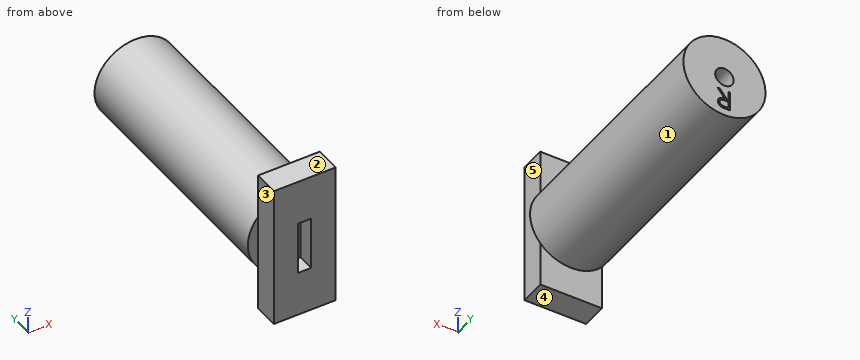
from build123d import *

# Parameters (mm, degrees)
SKETCH1_R           = 10
BOSS_EXTRUDE1_DEPTH = 4
SKETCH2_R           = 10
SKETCH2_R_2         = 8
SKETCH2_R_3         = 3.5
BOSS_EXTRUDE2_DEPTH = 52
SKETCH3_R           = 10
BOSS_EXTRUDE3_DEPTH = 4
CUT_EXTRUDE1_DEPTH  = 2
SKETCH5_R           = 2.25
CUT_EXTRUDE2_DEPTH  = 50
SKETCH6_W           = 15
SKETCH6_H           = 35
BOSS_EXTRUDE4_DEPTH = 6.18
SKETCH7_W           = 3.18
SKETCH7_H           = 13
CUT_EXTRUDE3_DEPTH  = 4.18


with BuildPart() as part:
    # Sketch1 → Boss-Extrude1 (new body)
    with BuildSketch(Plane(origin=(0, 0, 0), x_dir=(1, 0, 0), z_dir=(0, 1, 0))):
        with Locations(Location((0, 0, 0), (0, 0, 270))):
            Circle(SKETCH1_R)
    extrude(amount=BOSS_EXTRUDE1_DEPTH)

    # Sketch2 → Boss-Extrude2 (add)
    # profile 1 of 2: a face of its own
    with BuildSketch(Plane(origin=(0, 4, 0), x_dir=(1, 0, 0), z_dir=(0, 1, 0))):
        with Locations(Location((0, 0, 0), (0, 0, 270))):
            Circle(SKETCH2_R)
        with Locations(Location((0, 0, 0), (0, 0, 90))):
            Circle(SKETCH2_R_2, mode=Mode.SUBTRACT)
    # profile 2 of 2: a face of its own
    with BuildSketch(Plane(origin=(0, 4, 0), x_dir=(1, 0, 0), z_dir=(0, 1, 0))):
        with Locations(Location((0, 0, 0), (0, 0, 90))):
            Circle(SKETCH2_R_3)
    extrude(amount=BOSS_EXTRUDE2_DEPTH)

    # Sketch3 → Boss-Extrude3 (add)
    with BuildSketch(Plane(origin=(0, 56, 0), x_dir=(1, 0, 0), z_dir=(0, 1, 0))):
        with Locations(Location((0, 0, 0), (0, 0, 270))):
            Circle(SKETCH3_R)
    extrude(amount=BOSS_EXTRUDE3_DEPTH)

    # Sketch4 → Cut-Extrude1 (cut)
    with BuildSketch(Plane(origin=(0, 60, 0), x_dir=(1, 0, 0), z_dir=(0, 1, 0))):
        with BuildLine():
            Line((-1.404326923, 8.220249015), (-0.451254507, 8.220249015))
            add(Edge.make_bspline(
                [(-0.451254507, 8.220249015), (-0.387653186, 8.220037307), (-0.265531604, 8.219630804), (-0.090580118, 8.217364176), (0.068388182, 8.210867642), (0.211290178, 8.205277034), (0.338123247, 8.195082643), (0.449276311, 8.185339048), (0.544237428, 8.172584174), (0.601721961, 8.16073858), (0.627749399, 8.155375217)],
                knots=[0, 0, 0, 0, 1.410062039, 2.707475311, 3.878576406, 4.937260626, 5.877586885, 6.699081471, 7.410979367, 8, 8, 8, 8], degree=3))
            add(Edge.make_bspline(
                [(0.627749399, 8.155375217), (0.662592698, 8.146766297), (0.731535995, 8.129732108), (0.830800192, 8.093728152), (0.925389325, 8.052063591), (1.014910479, 8.003127243), (1.098915252, 7.946555846), (1.178269811, 7.883326008), (1.253334245, 7.813783703), (1.32107282, 7.73617558), (1.384943458, 7.654755186), (1.438812268, 7.56671186), (1.485248657, 7.474643853), (1.522219967, 7.377614831), (1.551989638, 7.276565777), (1.572980343, 7.170581378), (1.585568566, 7.06014448), (1.586850162, 6.984818183), (1.5875, 6.946623714)],
                knots=[0, 0, 0, 0, 1.027469482, 2.033020251, 3.019912614, 3.986113645, 4.951240523, 5.91722682, 6.890402269, 7.87763091, 8.8651537, 9.85103654, 10.82876324, 11.815024772, 12.821070561, 13.842952187, 14.906261191, 16, 16, 16, 16], degree=3))
            add(Edge.make_bspline(
                [(1.5875, 6.946623714), (1.585501113, 6.883166661), (1.581600768, 6.759345515), (1.545235537, 6.579648387), (1.485668201, 6.412022927), (1.40358544, 6.256680195), (1.299056082, 6.116648209), (1.17342842, 5.993652625), (1.02663237, 5.890728316), (0.889976765, 5.819355035), (0.769262086, 5.773644684), (0.669884614, 5.741482353), (0.56148062, 5.716633036), (0.445088747, 5.694371571), (0.32022463, 5.677564444), (0.187187541, 5.665254614), (0.045882599, 5.657561069), (-0.051189492, 5.656415341), (-0.101126803, 5.655825938)],
                knots=[0, 0, 0, 0, 1.260483769, 2.459530307, 3.627416485, 4.787058657, 5.939039949, 7.08810263, 8.267026773, 9.491475466, 10.141966685, 10.831826277, 11.566392101, 12.351337768, 13.187381173, 14.07005841, 15.007169909, 16, 16, 16, 16], degree=3))
            Line((-0.101126803, 5.655825938), (1.648557692, 3.457749015))
            Line((1.648557692, 3.457749015), (1.120027043, 3.457749015))
            Line((1.120027043, 3.457749015), (-0.629657452, 5.655825938))
            Line((-0.629657452, 5.655825938), (-0.976923077, 5.655825938))
            Line((-0.976923077, 5.655825938), (-0.976923077, 3.457749015))
            Line((-0.976923077, 3.457749015), (-1.404326923, 3.457749015))
            Line((-1.404326923, 3.457749015), (-1.404326923, 8.220249015))
        make_face()
        with BuildLine():
            Line((-0.976923077, 7.731787476), (-0.976923077, 6.144287476))
            Line((-0.976923077, 6.144287476), (-0.104942909, 6.137609291))
            add(Edge.make_bspline(
                [(-0.104942909, 6.137609291), (-0.064230284, 6.13759128), (0.014682377, 6.137556369), (0.128847211, 6.142990757), (0.235146363, 6.149172915), (0.333173243, 6.158628989), (0.422971644, 6.170815644), (0.504496681, 6.186059705), (0.577881434, 6.203819833), (0.663468374, 6.231308474), (0.759040225, 6.27485952), (0.862905533, 6.338221859), (0.951355143, 6.417917696), (1.026082663, 6.509049435), (1.08613021, 6.60924733), (1.128464827, 6.717310318), (1.15532865, 6.830510314), (1.158497136, 6.908313383), (1.160096154, 6.947577741)],
                knots=[0, 0, 0, 0, 1.146690395, 2.22261258, 3.21895312, 4.145990853, 4.996080663, 5.770904154, 6.481378293, 7.121626537, 8.300444488, 9.431385265, 10.535395872, 11.636531494, 12.74115979, 13.810798291, 14.895190096, 16, 16, 16, 16], degree=3))
            add(Edge.make_bspline(
                [(1.160096154, 6.947577741), (1.158460411, 6.985877186), (1.155218964, 7.061772711), (1.128754747, 7.172883074), (1.084001696, 7.277749174), (1.023691794, 7.37594442), (0.950214372, 7.46507901), (0.86405692, 7.541343172), (0.767575208, 7.60427548), (0.677399041, 7.644490547), (0.596798202, 7.66914649), (0.526817129, 7.686497181), (0.447744011, 7.700436976), (0.359194905, 7.711605802), (0.261547829, 7.721205566), (0.15430905, 7.727671379), (0.038190074, 7.731500244), (-0.042292, 7.731689504), (-0.083954327, 7.731787476)],
                knots=[0, 0, 0, 0, 1.101028733, 2.181837193, 3.264309656, 4.369019818, 5.486613113, 6.575447106, 7.666700264, 8.788928104, 9.402425223, 10.0903467, 10.862060571, 11.710948788, 12.657782767, 13.684531032, 14.801375019, 16, 16, 16, 16], degree=3))
            Line((-0.083954327, 7.731787476), (-0.976923077, 7.731787476))
        make_face(mode=Mode.SUBTRACT)
    extrude(amount=-CUT_EXTRUDE1_DEPTH, mode=Mode.SUBTRACT)

    # Sketch5 → Cut-Extrude2 (cut)
    with BuildSketch(Plane(origin=(0, 60, 0), x_dir=(1, 0, 0), z_dir=(0, 1, 0))):
        with Locations(Location((0, 0, 0), (0, 0, 270))):
            Circle(SKETCH5_R)
    extrude(amount=-CUT_EXTRUDE2_DEPTH, mode=Mode.SUBTRACT)

    # Sketch6 → Boss-Extrude4 (add)
    with BuildSketch(Plane.XZ):
        Rectangle(SKETCH6_W, SKETCH6_H)
    extrude(amount=BOSS_EXTRUDE4_DEPTH)

    # Sketch7 → Cut-Extrude3 (cut)
    with BuildSketch(Plane.XZ.offset(6.18)):
        Rectangle(SKETCH7_W, SKETCH7_H)
    extrude(amount=-CUT_EXTRUDE3_DEPTH, mode=Mode.SUBTRACT)


solid = part.part
Check sheet for the modelled part. Datum: model origin and axes. Units: mm. Face numbers are marked on the shaded views. A direction names the side the tool comes from. Coordinates: 2 decimals unless noted, no trailing zeros. Write each loop counter-clockwise with the first axis right and the second up, starting at its lowest first coordinate (ties: lowest second). Pieces come first, ordered by that corner, then holes. Notation, with made-up numbers: M 22.5,82 L 69.5,82 A12 cw 69.5,88 Z; hole C 29.25,86.5 d5. An arc over 180 degrees is marked long. Answer as CSV lines item,"result".
Q1. Set-up check for the marked faces 4 and 5: record each of +Z, -Z, +X, -X, +Y, -Y from which the full face is reachable in a straight line by a thin tool's end or side.
Check result:
face 4,"-Z, +X, -X, +Y, -Y"
face 5,"+Z, -Z, +X, -Y"
Q2. Cross-section at C-C (y = 5). Record the boundary of the cut face in (x, z).
Check result:
outline,"C 0,0 d20; C 0,0 d7; hole C 0,0 d16"
Q3. Go/stop test with flat-tipped pins: pin 1 (3 mm diameter, centred on x = -3.5, z = 12.5, fed in from +Y); pin 2 (2 mm diameter, centred on x = 1, z = 0.5, fed in from +Y); pin 3 (2 mm diameter, centred on y = 59, z = -4.5, fed in from -X); pin 4 (1.5 mm diameter, centred on y = 34, z = 12, fed in from -X). Record where each tip stops, or that it passes through.
Check result:
pin 1,"y = 0"
pin 2,"y = 10"
pin 3,"x = -9.37"
pin 4,"through"
Q4. Material ranges on probe 1 along X at (y, z) = (34, 0); probe 2 along Y at (x, z) = (2.25, -5); probe 3 along Y at (x, z) = (0.5, -5), recorded low to high. Write a range as from..to.
Check result:
probe 1,"-10..-8, -3.5..-2.25, 2.25..3.5, 8..10"
probe 2,"-6.18..4, 56..60"
probe 3,"-2..4, 56..60"
Q5. Cross-section at A-A (z = 0). Record the boundary of the cut face in (x, y).
Check result:
outline,"M -10,0 L -7.5,0 L -7.5,-6.18 L -1.59,-6.18 L -1.59,-2 L 1.59,-2 L 1.59,-6.18 L 7.5,-6.18 L 7.5,0 L 10,0 L 10,60 L 2.25,60 L 2.25,10 L -2.25,10 L -2.25,60 L -10,60 Z; hole M -8,4 L -3.5,4 L -3.5,56 L -8,56 Z; hole M 3.5,4 L 8,4 L 8,56 L 3.5,56 Z"
Q6. Mould release check, pull along Z, two halves, no side actions. Record for the marked faces 1, 2 and 3: released by +Z, released by -Z, zero draft, split by the parting line, or undercut.
Check result:
face 1,"split by the parting line"
face 2,"released by +Z"
face 3,"zero draft"
Q7. Cross-section at D-D (z = -14.5). Record the boundary of the cut face in (x, y), then the cut area to 3 significant figures.
Check result:
outline,"M -7.5,-6.18 L 7.5,-6.18 L 7.5,0 L -7.5,0 Z"
area,"92.7 mm^2"
Q8. Cross-section at B-B (y = 30). Record the boundary of the cut face in (x, z), then the cut area to 3 significant figures.
Check result:
outline,"C 0,0 d20; C 0,0 d7; hole C 0,0 d16; hole C 0,0 d4.5"
area,"136 mm^2"
